```python
from build123d import *

# Parameters (mm, degrees)
F0_W     = 14.6975922398
F0_H     = 32.3806256056
F1_DEPTH = 8.382


with BuildPart() as f1:
    # F0 (on Right) → F1 (new body)
    with BuildSketch(Plane.YZ):
        Polygon((26.4097284526, 29.4411070645), (20.163256675, 32.3806256056), (20.163256675, 0), (26.4097284526, 0), align=None)
        Polygon((5.4656644352, 0), (5.4656644352, 32.3806256056), (0, 29.4411070645), (0, 0), align=None)
        with Locations((12.8144605551, 16.1903128028)):
            Rectangle(F0_W, F0_H)
    extrude(amount=-F1_DEPTH)


solid = f1.part
```
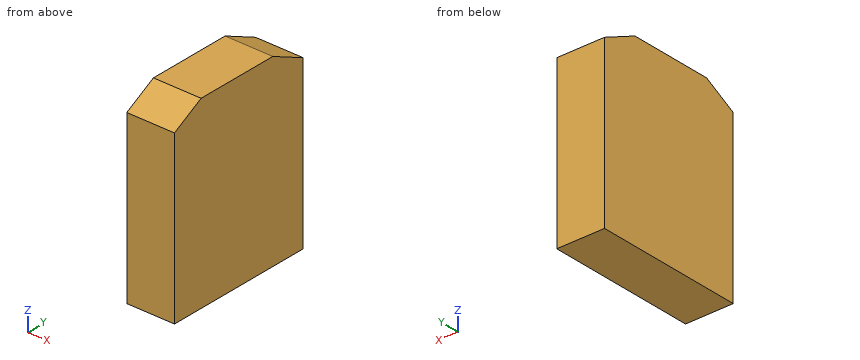
Could you check a few things on this model? Use its own coordinates, in mm. Give positions to 0.01 mm unless a question says otherwise; leave off trailing zeros. Write each loop counter-clockwise with the first axis right and the second up, starting at its lowest first coordinate (ties: lowest second). Pieces come first, ordered by that corner, then holes. Notation, with made-up numbers: (26, -34.5) - (30, -34.5) arc R31 ccw to (30, -7.5) - close; hole circle Ø5 at (-12, 73.25). An arc over 180 degrees is marked (long way). One line per item, written item: value. Start each with the question number.
Item 1: Please list where these lines run through material, in increasing order: line 1 (Z direction, x = -4.5, y = 22.75); line 2 (Z direction, x = -1.5, y = 3.75); line 3 (Y direction, x = -4.75, z = 30). Write a range as from..to.
Item 2: Imagine slicing it at A-A, the plane x = -7.25. List the corners of the cut face in (y, z) for me.
Item 3: I'm going to push a flat-ended pin straight in: pin 1 (4 mm diameter, centred on x = -7, y = 22.5, fed in from +Z). Where does the tip first touch, or does it pass through?
Item 4: Imagine slicing it at C-C, the plane y = 3.5. List the corners of the cut face in (x, z) for me, and give its area (3 significant figures).
Item 5: Imagine slicing it at B-B, the plane y = 22.75. List the corners of the cut face in (x, z) for me.
Geometry says:
1. line 1: 0..31.16
1. line 2: 0..31.46
1. line 3: 1.04..25.22
2. outline: (0, 0) - (26.41, 0) - (26.41, 29.44) - (20.16, 32.38) - (5.47, 32.38) - (0, 29.44) - close
3. pin 1: z = 32.22
4. outline: (-8.38, 0) - (0, 0) - (0, 31.32) - (-8.38, 31.32) - close
4. area: 263 mm^2
5. outline: (-8.38, 0) - (0, 0) - (0, 31.16) - (-8.38, 31.16) - close
